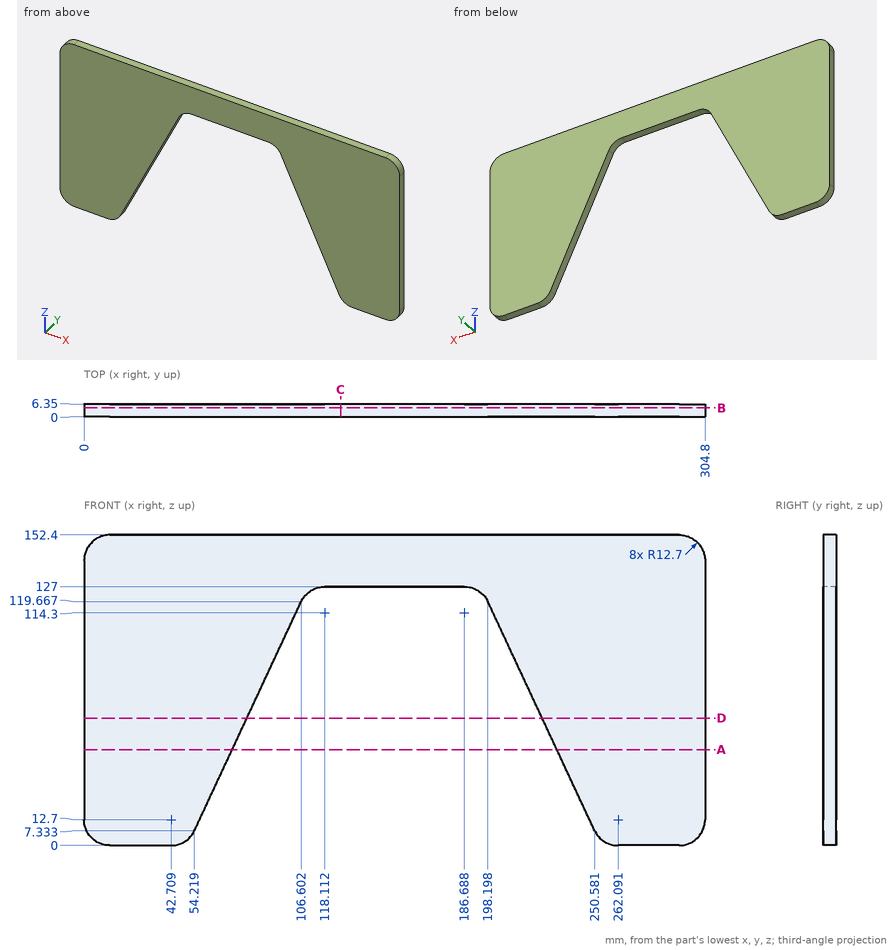
Part print with two shaded views. Sizes in mm from the minimum x, y, z corner. Round coordinates to 2 decimals unless told otherwise and drop trailing zeros. Order: outer loops, then holes, each group sorted by start corner. A loop starts at its lowest first (then second) coordinate and runs counter-clockwise, first axis right, second up. Notation, with made-up numbers: (36.25, 81.5) - (71.25, 81.5) arc R21 cw to (71.25, 102.5) - close; hole circle Ø11 at (79.5, 44). An arc over 180 degrees is marked (long way). Answer as CSV lines item,"result". Start each with the question number.
1. Saw through at B-B, the plane y = 4.5. Write the cut outline in (x, z).
2. Saw through at A-A, the plane z = 47. Write the cut outline in (x, y).
3. Saw through at D-D, the plane z = 62.5. Write the cut outline in (x, y).
4. Drill centre lines: L1, parallel to Z at x = 165, y = 3.25; L2, parallel to X at y = 5.25, z = 61 (1 decimal); L3, parallel to X at y = 2, z = 37. Where is each one in solid material? Low to high. Write a range as [from, to].
5. Saw through at C-C, the plane x = 126. Write the cut outline in (y, z), and give its area (3 significant figures).
6. Pin check, flat tips, straight feed: pin 1 (5 mm diameter, centred on x = 73.5, z = 105.5, fed in from -Y); pin 2 (3 mm diameter, centred on x = 140.5, y = 2, fed in from -Z). Stop position of each tip, or through.
Model answer:
1,outline,"(0, 12.7) arc R12.7 ccw to (12.7, 0) - (42.71, 0) arc R12.7 ccw to (54.22, 7.33) - (106.6, 119.67) arc R12.7 cw to (118.11, 127) - (186.69, 127) arc R12.7 cw to (198.2, 119.67) - (250.58, 7.33) arc R12.7 ccw to (262.09, 0) - (292.1, 0) arc R12.7 ccw to (304.8, 12.7) - (304.8, 139.7) arc R12.7 ccw to (292.1, 152.4) - (12.7, 152.4) arc R12.7 ccw to (0, 139.7) - close"
2,outline,"(0, 0) - (72.72, 0) - (72.72, 6.35) - (0, 6.35) - close; (232.08, 0) - (304.8, 0) - (304.8, 6.35) - (232.08, 6.35) - close"
3,outline,"(0, 0) - (79.94, 0) - (79.94, 6.35) - (0, 6.35) - close; (224.86, 0) - (304.8, 0) - (304.8, 6.35) - (224.86, 6.35) - close"
4,L1,"z = [127, 152.4]"
4,L2,"x = [0, 79.2], [225.6, 304.8]"
4,L3,"x = [0, 68.05], [236.75, 304.8]"
5,outline,"(0, 127) - (6.35, 127) - (6.35, 152.4) - (0, 152.4) - close"
5,area,"161 mm²"
6,pin 1,"stops at y = 0"
6,pin 2,"stops at z = 127"
